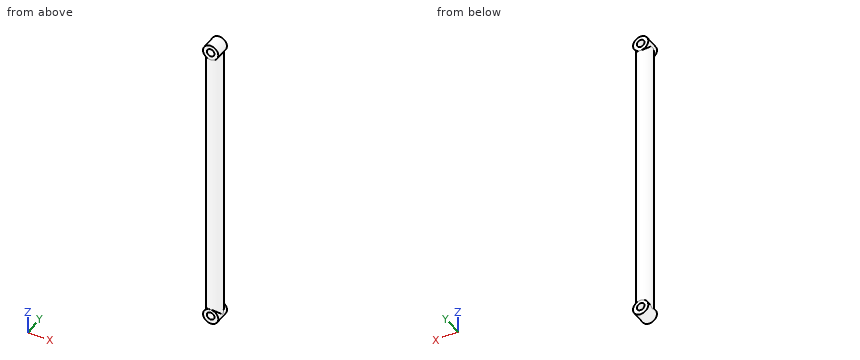
from build123d import *

# Parameters (mm, degrees)
SKIZZE1_R                       = 2
AUFSATZ_LINEAR_AUSTRAGEN1_DEPTH = 75
AUFSATZ_LINEAR_START            = 2
SKIZZE2_R                       = 2
AUFSATZ_LINEAR_AUSTRAGEN2_DEPTH = 4
SKIZZE3_R                       = 1
SCHNITT_LINEAR_AUSTRAGEN1_DEPTH = 4


with BuildPart() as part:
    # Skizze1 → Aufsatz-Linear austragen1 (new body)
    with BuildSketch(Plane.XY):
        Circle(SKIZZE1_R)
    extrude(amount=AUFSATZ_LINEAR_AUSTRAGEN1_DEPTH)

    # Skizze2 → Aufsatz-Linear austragen2 (add)
    with BuildSketch(Plane(origin=(0, 0, 0), x_dir=(1, 0, 0), z_dir=(0, 1, 0)).offset(AUFSATZ_LINEAR_START)):
        with Locations((0, -75.688838901)):
            Circle(SKIZZE2_R)
        with Locations((0, 0.161056254)):
            Circle(SKIZZE2_R)
    extrude(amount=-AUFSATZ_LINEAR_AUSTRAGEN2_DEPTH)

    # Skizze3 → Schnitt-Linear austragen1 (cut)
    with BuildSketch(Plane(origin=(0, 2, 0), x_dir=(1, 0, 0), z_dir=(0, 1, 0))):
        with Locations((0, -75.688838901)):
            Circle(SKIZZE3_R)
        Circle(SKIZZE3_R)
    extrude(amount=-SCHNITT_LINEAR_AUSTRAGEN1_DEPTH, mode=Mode.SUBTRACT)


solid = part.part
Model file for the job. Use its own axes, mm. Coordinates: 2 decimals unless noted, no trailing zeros. Write each loop counter-clockwise with the first axis right and the second up, starting at its lowest first coordinate (ties: lowest second). Pieces come first, ordered by that corner, then holes. Notation, with made-up numbers: (41, -36.5) - (88, -36.5) arc R29 ccw to (88, -0.5) - close; hole circle Ø8 at (-4, -15). An arc over 180 degrees is marked (long way). Write each question's results on one line, items separated by ' | '. Start each with the question number.
1) Probe line 1 along Z through (x, y) = (0, 0.25); line 2 along X through (y, z) = (-0.5, 0); line 3 along Z through (x, y) = (0.55, 0.95). List the from-to ranges inside material, lowest first. Write a range as from..to.
2) Flat gauge pins, fed straight in: P1, Ø1.5, axis at y = -0.5, z = 58.5, coming from the -X side; P2, Ø1.5, axis at y = 1, z = 23.5, coming from the +X side. Where does each tip first touch, or does it go through?
3) Cut at A-A (z = 21). Write the cut outline in (x, y), then the cut area to 3 significant figures.
Returned:
1) line 1: -2.16..-1, 1..74.69, 76.69..77.69 | line 2: -1.99..-1, 1..1.99 | line 3: -2.08..-0.84, 0.84..74.85, 76.52..77.61
2) P1: x = -2 | P2: x = 1.98
3) outline: circle Ø4 at (0, 0) | area: 12.6 mm^2
